```python
from build123d import *

# Parameters (mm, degrees)
SKETCH_1_W      = 74.4
SKETCH_1_H      = 44.02
SKETCH_1_R      = 1.6
EXTRUDE_1_DEPTH = 2
SKETCH_2_W      = 61.56
SKETCH_2_H      = 42.9
EXTRUDE_2_DEPTH = 5
SKETCH_3_W      = 7.8
SKETCH_3_H      = 15.12
EXTRUDE_3_DEPTH = 9


with BuildPart() as part:
    # 草图1 → 凸台-拉伸1 (new body)
    with BuildSketch(Plane(origin=(0, 0, 0), x_dir=(1, 0, 0), z_dir=(0, 1, 0))):
        Rectangle(SKETCH_1_W, SKETCH_1_H)
        with Locations(Location((-34, 18.25, 0), (0, 0, 270))):
            Circle(SKETCH_1_R, mode=Mode.SUBTRACT)
        with Locations(Location((34, 18.25, 0), (0, 0, 90))):
            Circle(SKETCH_1_R, mode=Mode.SUBTRACT)
        with Locations(Location((34, -18.25, 0), (0, 0, 270))):
            Circle(SKETCH_1_R, mode=Mode.SUBTRACT)
        with Locations(Location((-34, -18.25, 0), (0, 0, 90))):
            Circle(SKETCH_1_R, mode=Mode.SUBTRACT)
    extrude(amount=EXTRUDE_1_DEPTH)

    # 草图2 → 凸台-拉伸2 (add)
    with BuildSketch(Plane(origin=(0, 2, 0), x_dir=(1, 0, 0), z_dir=(0, 1, 0))):
        Rectangle(SKETCH_2_W, SKETCH_2_H)
    extrude(amount=EXTRUDE_2_DEPTH)

    # 草图3 → 凸台-拉伸3 (add)
    with BuildSketch(Plane.XZ):
        with Locations((33.3, 0)):
            Rectangle(SKETCH_3_W, SKETCH_3_H)
    extrude(amount=EXTRUDE_3_DEPTH)


solid = part.part
```
Source: CAD feature listing. Evaluate the final solid. Frame: model axes, mm. A direction names the side the tool comes from. Give positions to 0.01 mm unless a question says otherwise; leave off trailing zeros. Order: outer loops, then holes, each group sorted by start corner. A loop starts at its lowest first (then second) coordinate and runs counter-clockwise, first axis right, second up.
(1) Material intervals for line 1 along X through (y, z) = (1.1, -18.25); line 2 along Y through (x, z) = (31.5, 15); line 3 along Y through (x, z) = (-17, 11), sorted ascending.
(2) Pull-direction query (Z, two-part tool) for faces 1 (the face through (33, -4, 7.56)), 2 (the face through (-33, 2, 0)), 3 (the face through (-35.56, 0.99, -18.6)); classes: +Z half, -Z half, draft (parallel to the pull), parting line (faces both ways), or undercut.
(3) Section query C-C (z = -4). Return the cut outline in (x, y), plus the area to 3 significant figures.
(4) Contact query for flat-ended pins moving along their axis: P1, Ø3.5, axis at x = -34, z = -18.25, coming from the -Y side; P2, Ø2.5, axis at y = 4.5, z = -2.5, coming from the +X side; P3, Ø7, axis at y = -5, z = 2, coming from the -X side. Output: stop coordinate, or through.
(5) Access query for faces 4 (the face through (33, -4, -7.56)), 5 (the face through (30.78, 4, 0)), 6 (the face through (29.4, -4, 0)). Directions: +Z, -Z, +X, -X, +Y, -Y. A direction counts if a zero-diameter tool reaches every point of the face in a straight line with its end or side. Return the directions, or none.
(6) Section query A-A (z = -18.25). Return the cut outline in (x, y), plus the area to 3 significant figures.
(7) Section query B-B (x = 34). Return the cut outline in (y, z).
(8) Section query D-D (x = -34). Return the cut outline in (y, z), plus the area to 3 significant figures.
Outcome:
1. line 1: x = -37.2 to -35.6, -32.4 to 32.4, 35.6 to 37.2
1. line 2: y = 0 to 2
1. line 3: y = 0 to 7
2. face 1: +Z half
2. face 2: draft
2. face 3: undercut
3. outline: (-37.2, 0) - (29.4, 0) - (29.4, -9) - (37.2, -9) - (37.2, 2) - (30.78, 2) - (30.78, 7) - (-30.78, 7) - (-30.78, 2) - (-37.2, 2) - close
3. area: 527 mm2
4. P1: stops at y = 0
4. P2: stops at x = 30.78
4. P3: stops at x = 29.4
5. face 4: -Z, +X, -X, -Y
5. face 5: +Z, -Z, +X, +Y
5. face 6: +Z, -Z, -X, -Y
6. outline: (-37.2, 0) - (-35.6, 0) - (-35.6, 2) - (-37.2, 2) - close; (-32.4, 0) - (32.4, 0) - (32.4, 2) - (30.78, 2) - (30.78, 7) - (-30.78, 7) - (-30.78, 2) - (-32.4, 2) - close; (35.6, 0) - (37.2, 0) - (37.2, 2) - (35.6, 2) - close
6. area: 444 mm2
7. outline: (-9, -7.56) - (0, -7.56) - (0, -16.65) - (2, -16.65) - (2, 16.65) - (0, 16.65) - (0, 7.56) - (-9, 7.56) - close; (0, -22.01) - (2, -22.01) - (2, -19.85) - (0, -19.85) - close; (0, 19.85) - (2, 19.85) - (2, 22.01) - (0, 22.01) - close
8. outline: (0, -22.01) - (2, -22.01) - (2, -19.85) - (0, -19.85) - close; (0, -16.65) - (2, -16.65) - (2, 16.65) - (0, 16.65) - close; (0, 19.85) - (2, 19.85) - (2, 22.01) - (0, 22.01) - close
8. area: 75.2 mm2
